Input: part model. Units: mm. Frame: model coordinates. Coordinates: 2 decimals unless noted, no trailing zeros. Loops run counter-clockwise (first coordinate to the right, second up) from the corner with the lowest first, then second, coordinate; pieces in that order, holes last. Notation, with made-up numbers: (16, -11.75) - (57, -11.75) arc R30 ccw to (57, 26.25) - close; hole circle Ø2 at (12.25, 69.5). An arc over 180 degrees is marked (long way). Answer as CSV lines item,"result". Start each with the question number.
```python
from build123d import *

# Parameters (mm, degrees)
F0_W     = 85.746526
F0_H     = 100
F0_R     = 7.66167
F0_R_2   = 8
F1_DEPTH = 100


with BuildPart() as f1:
    # F0 (on Front) → F1 (new body)
    with BuildSketch(Plane.XZ):
        Rectangle(F0_W, F0_H)
        with Locations((-31.075926, -17.983756)):
            Circle(F0_R, mode=Mode.SUBTRACT)
        with Locations((11.22186, 24.60177)):
            Circle(F0_R_2, mode=Mode.SUBTRACT)
        Polygon((-42.873263, 50), (42.873263, 50), (25.608866, 60.070896), (23.594683, 77.047562), align=None)
    extrude(amount=F1_DEPTH)


solid = f1.part
```
Item 1: Contact query for a flat-ended pin moving along its axis: P1, Ø5, axis at x = 10.5, y = -23, coming from the +Z side. Output: stop coordinate, or through.
Item 2: Section query C-C, the plane x = -9.5. Output: boundary loops of the cut face in (y, z), and give its area (3 significant figures).
Item 3: Material intervals for probe 1 along Z at (x, y) = (-26, -61); probe 2 along Z at (x, y) = (15, -11.5); probe 3 along Z at (x, y) = (2, -90), sorted ascending.
Item 4: Section query D-D, the plane z = 69. Output: boundary loops of the cut face in (x, y), and give its area (3 significant figures).
Item 5: Draft query along Z for faces 1 (the flat face through (42.873, -49, -1)), 2 (the cylindrical face through (10.18, -49.3, 32.534)), 3 (the flat face through (-1, -49, -50)). Return one class per face: pulls with the +Z half, pulls with the -Z half, needs draft (parallel to the pull), parting line crosses it, or undercut.
Item 6: Section query B-B, the plane y = -54. Output: boundary loops of the cut face in (x, z).
Item 7: Section query A-A, the plane z = -22. Output: boundary loops of the cut face in (x, y), and give its area (3 significant figures).
Response values:
1,P1,"stops at z = 72.74"
2,outline,"(-100, -50) - (0, -50) - (0, 63.58) - (-100, 63.58) - close"
2,area,"11,400 mm²"
3,probe 1,"z = -50 to -23.72, -12.24 to 56.87"
3,probe 2,"z = -50 to 17.55, 31.65 to 73.55"
3,probe 3,"z = -50 to 68.26"
4,outline,"(3.82, -100) - (24.55, -100) - (24.55, 0) - (3.82, 0) - close"
4,area,"2,070 mm²"
5,face 1,"needs draft"
5,face 2,"undercut"
5,face 3,"pulls with the -Z half"
6,outline,"(-42.87, -50) - (42.87, -50) - (42.87, 50) - (25.61, 60.07) - (23.59, 77.05) - (-42.87, 50) - close; hole circle Ø15.32 at (-31.08, -17.98); hole circle Ø16 at (11.22, 24.6)"
7,outline,"(-42.87, -100) - (-37.6, -100) - (-37.6, 0) - (-42.87, 0) - close; (-24.55, -100) - (42.87, -100) - (42.87, 0) - (-24.55, 0) - close"
7,area,"7,270 mm²"
